Part model, mm, in its own coordinate system. Face numbers are marked on the shaded views. A direction names the side the tool comes from. Round coordinates to 2 decimals unless told otherwise and drop trailing zeros. Write each loop counter-clockwise with the first axis right and the second up, starting at its lowest first coordinate (ties: lowest second). Pieces come first, ordered by that corner, then holes.
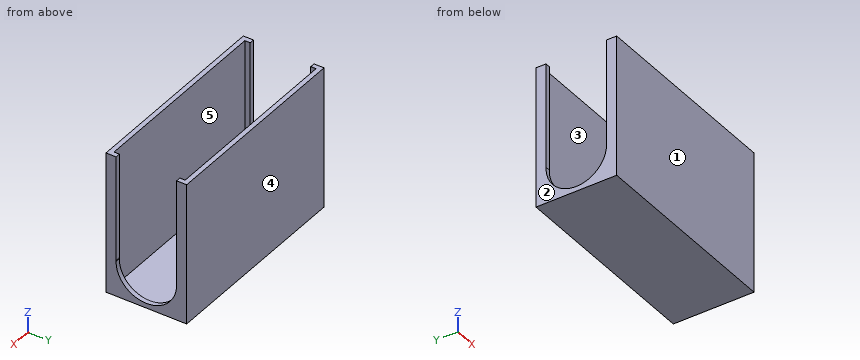
from build123d import *

# Parameters (mm, degrees)
F0_W     = 63.5
F0_H     = 25.4
F1_DEPTH = 44.45
F2_T     = -1.5
F4_DEPTH = 1.5


# Not quite as in the source:
# - a pattern or mirror of a feature is missing from the dataset's text; its kind, count and spacing are read off the source's solid


with BuildPart() as f1:
    # F0 (on Top) → F1 (new body)
    with BuildSketch(Plane.XY):
        Rectangle(F0_W, F0_H)
    extrude(amount=F1_DEPTH)

    # F2
    f2_openings = [f1.faces().sort_by_distance(p)[0] for p in [
        (0, 0, 44.45),
    ]]
    offset(amount=F2_T, openings=f2_openings)

    # F3 (on face) → F4 (cut)
    with BuildSketch(Plane(origin=(-31.75, 0, 0), x_dir=(0, -1, 0), z_dir=(-1, 0, 0))):
        with BuildLine():
            Line((-9.5163858686, 11.43), (9.5163858686, 11.43))
            ThreePointArc((9.5163858686, 11.43), (0, 20.55), (-9.5163858686, 11.43))
        make_face()
        with BuildLine():
            ThreePointArc((-9.5163858686, 11.43), (-0.2025457993, 1.5021537764), (9.525, 11.025))
            ThreePointArc((9.525, 11.025), (9.5228462236, 11.2275457993), (9.5163858686, 11.43))
            Line((9.5163858686, 11.43), (-9.5163858686, 11.43))
        make_face()
        with BuildLine():
            ThreePointArc((-9.5163858686, 11.43), (0, 20.55), (9.5163858686, 11.43))
            Line((9.5163858686, 11.43), (9.5163858686, 44.45))
            Line((9.5163858686, 44.45), (-9.5336141314, 44.45))
            Line((-9.5336141314, 44.45), (-9.5336141314, 11.43))
            Line((-9.5336141314, 11.43), (-9.5163858686, 11.43))
        make_face()
    f4 = extrude(amount=-F4_DEPTH, mode=Mode.SUBTRACT)

    # F4_copies: F4 across plane
    add(f4.mirror(Plane(origin=(0, 0, 0), x_dir=(0, 0, 1), z_dir=(1, 0, 0))), mode=Mode.SUBTRACT)


solid = f1.part
Q1. Wall check: line 1 (Y direction, x = -21.5, z = 16); line 2 (X direction, y = 10.25, z = 12); line 3 (Z direction, x = 8.5, y = 8.5). Give the ranges that are in metal, low to high.
Q2. Saw through at A-A, the plane z = 35.5. Write the cut outline in (x, y), and give its area (3 significant figures).
Q3. Tool access for the marked faces 4 and 5: list every direction of +Z, -Z, +X, -X, +Y, -Y with a clear straight run to the whole face (end or side of a thin tool).
Q4. Saw through at D-D, the plane y = 5.5. Write the cut outline in (x, z).
Q5. Saw through at C-C, the plane z = 6.5. Write the cut outline in (x, y), and give its area (3 significant figures).
Q6. Saw through at B-B, the plane x = -17. Write the cut outline in (y, z), and give its area (3 significant figures).
Q7. Two-plate mould, pull along Y, no slides. Class the marked faces 1, 2 and 3: released by +Y, released by -Y, zero draft, split by the parting line, or undercut.
Q8. Drop flat-ended pins along their axis: P1, Ø3.5, axis at y = 6.5, z = 13.5, coming from the -X side; P2, Ø5, axis at x = -6.5, y = -6, coming from the +Z side. Give the stop position or say it passes through.
Computed:
1. line 1: y = -12.7 to -11.2, 11.2 to 12.7
1. line 2: x = -31.75 to -30.25, 30.25 to 31.75
1. line 3: z = 0 to 1.5
2. outline: (-31.75, -12.7) - (31.75, -12.7) - (31.75, -9.52) - (30.25, -9.52) - (30.25, -11.2) - (-30.25, -11.2) - (-30.25, -9.52) - (-31.75, -9.52) - close; (-31.75, 9.53) - (-30.25, 9.53) - (-30.25, 11.2) - (30.25, 11.2) - (30.25, 9.53) - (31.75, 9.53) - (31.75, 12.7) - (-31.75, 12.7) - close
2. area: 201 mm2
3. face 4: +Z, -Z, +X, -X, +Y
3. face 5: +Z
4. outline: (-31.75, 0) - (31.75, 0) - (31.75, 3.25) - (30.25, 3.25) - (30.25, 1.5) - (-30.25, 1.5) - (-30.25, 3.25) - (-31.75, 3.25) - close
5. outline: (-31.75, -12.7) - (31.75, -12.7) - (31.75, -8.38) - (30.25, -8.38) - (30.25, -11.2) - (-30.25, -11.2) - (-30.25, -8.38) - (-31.75, -8.38) - close; (-31.75, 8.38) - (-30.25, 8.38) - (-30.25, 11.2) - (30.25, 11.2) - (30.25, 8.38) - (31.75, 8.38) - (31.75, 12.7) - (-31.75, 12.7) - close
5. area: 207 mm2
6. outline: (-12.7, 0) - (12.7, 0) - (12.7, 44.45) - (11.2, 44.45) - (11.2, 1.5) - (-11.2, 1.5) - (-11.2, 44.45) - (-12.7, 44.45) - close
6. area: 167 mm2
7. face 1: released by -Y
7. face 2: zero draft
7. face 3: undercut
8. P1: passes through
8. P2: stops at z = 1.5
